Part model, mm, in its own coordinate system. A direction names the side the tool comes from. Give positions to 0.01 mm unless a question says otherwise; leave off trailing zeros. Write each loop counter-clockwise with the first axis right and the second up, starting at its lowest first coordinate (ties: lowest second). Pieces come first, ordered by that corner, then holes. Notation, with made-up numbers: M 86,43 L 121,43 A21 cw 121,47 Z; hole C -38,31.25 d2. An arc over 180 degrees is marked long. Use CSV: the item, a comma, the result in double quotes. Start each with the question number.
1. 3-axis set-ups, long thin cutter, end or side, ignore diameter. For faces 1 (the face through (0, -15.875, 1)), 2 (the face through (9.525, 0, 1)): which of +Z, -Z, +X, -X, +Y, -Y reach the whole face in a straight line?
2. Mould opens along Y. For faces 3 (the face through (-7.9, -0.7, -19.1)), 4 (the face through (0, 19.05, 1)), 5 (the face through (0.154, 17.44, -2.053)) say: pulls with the +Y half, pulls with the -Y half, needs draft (parallel to the pull), parting line crosses it, or undercut.
3. Band-saw the part on A-A, the plane z = -5.55. List the corners of the cut face in (x, y) (3 decimals), then the cut area to 3 significant figures.
4. Band-saw the part on C-C, the plane y = 5.08. List the corners of the cut face in (x, z) (3 decimals), then the cut area to 3 significant figures.
5. Band-saw the part on D-D, the plane z = 13. List the corners of the cut face in (x, y) (3 decimals).
6. Drill centre lines: line 1 along Y through (x, z) = (4.5, -18) (3 decimals); line 2 along Y through (x, z) = (8.4, -26.67) (3 decimals); line 3 along X through (y, z) = (-14, 27.5) (3 decimals). Where is each one in solid material? Low to high. Write a range as from..to.
7. Band-saw the part on B-B, the plane x = 0. List the corners of the cut face in (y, z) (3 decimals), then the cut area to 3 significant figures.
from build123d import *

# Parameters (mm, degrees)
SKETCH1_W           = 19.05
SKETCH1_H           = 38.1
SKETCH1_W_2         = 12.7
SKETCH1_H_2         = 31.75
BOSS_EXTRUDE1_DEPTH = 44.45
SKETCH2_R           = 3.5
CUT_EXTRUDE1_DEPTH  = 76.2
SKETCH3_R           = 6.35
SKETCH3_R_2         = 9.525
CUT_EXTRUDE2_DEPTH  = 52.976990101


with BuildPart() as part:
    # Sketch1 → Boss-Extrude1 (new, symmetric)
    with BuildSketch(Plane.XY):
        Rectangle(SKETCH1_W, SKETCH1_H)
        Rectangle(SKETCH1_W_2, SKETCH1_H_2, mode=Mode.SUBTRACT)
    extrude(amount=BOSS_EXTRUDE1_DEPTH, both=True)

    # Sketch2 → Cut-Extrude1 (cut)
    with BuildSketch(Plane.XZ.offset(19.05)):
        with Locations(Location((0, 34.45, 0), (0, 0, 270))):
            Circle(SKETCH2_R)
        with Locations(Location((0, -5.55, 0), (0, 0, 270))):
            Circle(SKETCH2_R)
    extrude(amount=-CUT_EXTRUDE1_DEPTH, mode=Mode.SUBTRACT)

    # Sketch3 → Cut-Extrude2 (cut, through all)
    with BuildSketch(Plane(origin=(9.525, 0, 0), x_dir=(0, 0, -1), z_dir=(1, 0, 0))):
        with Locations((-21.59, 5.08)):
            Circle(SKETCH3_R)
        with Locations((26.67, 5.08)):
            Circle(SKETCH3_R_2)
    extrude(amount=-CUT_EXTRUDE2_DEPTH, mode=Mode.SUBTRACT)


solid = part.part
Output:
1,face 1,"+Z, -Z"
1,face 2,"+Z, -Z, +X, +Y, -Y"
2,face 3,"undercut"
2,face 4,"pulls with the +Y half"
2,face 5,"needs draft"
3,outline,"M -9.525,-19.05 L -3.5,-19.05 L -3.5,-15.875 L -6.35,-15.875 L -6.35,15.875 L -3.5,15.875 L -3.5,19.05 L -9.525,19.05 Z; M 3.5,-19.05 L 9.525,-19.05 L 9.525,19.05 L 3.5,19.05 L 3.5,15.875 L 6.35,15.875 L 6.35,-15.875 L 3.5,-15.875 Z"
3,area,"278 mm²"
4,outline,"M -9.525,-44.45 L -6.35,-44.45 L -6.35,-36.195 L -9.525,-36.195 Z; M -9.525,-17.145 L -6.35,-17.145 L -6.35,15.24 L -9.525,15.24 Z; M -9.525,27.94 L -6.35,27.94 L -6.35,44.45 L -9.525,44.45 Z; M 6.35,-44.45 L 9.525,-44.45 L 9.525,-36.195 L 6.35,-36.195 Z; M 6.35,-17.145 L 9.525,-17.145 L 9.525,15.24 L 6.35,15.24 Z; M 6.35,27.94 L 9.525,27.94 L 9.525,44.45 L 6.35,44.45 Z"
4,area,"363 mm²"
5,outline,"M -9.525,-19.05 L 9.525,-19.05 L 9.525,19.05 L -9.525,19.05 Z; hole M -6.35,-15.875 L 6.35,-15.875 L 6.35,15.875 L -6.35,15.875 Z"
6,line 1,"y = -19.05..-15.875, 15.875..19.05"
6,line 2,"y = -19.05..-4.445, 14.605..19.05"
6,line 3,"x = -9.525..-6.35, 6.35..9.525"
7,outline,"M -19.05,-44.45 L -15.875,-44.45 L -15.875,-9.05 L -19.05,-9.05 Z; M -19.05,-2.05 L -15.875,-2.05 L -15.875,30.95 L -19.05,30.95 Z; M -19.05,37.95 L -15.875,37.95 L -15.875,44.45 L -19.05,44.45 Z; M 15.875,-44.45 L 19.05,-44.45 L 19.05,-9.05 L 15.875,-9.05 Z; M 15.875,-2.05 L 19.05,-2.05 L 19.05,30.95 L 15.875,30.95 Z; M 15.875,37.95 L 19.05,37.95 L 19.05,44.45 L 15.875,44.45 Z"
7,area,"476 mm²"
